from build123d import *

# Parameters (mm, degrees)
F1_DEPTH  = 38
F3_DEPTH  = 25
F4_DEPTH  = 38
F0_W      = 25
F0_H      = 10
F5_DEPTH  = 5
F6_DEPTH  = 10
F7_DEPTH  = 15
F0_W_2    = 5
F0_H_2    = 5
F8_DEPTH  = 38
F0_H_3    = 23
F9_DEPTH  = 32
F11_DEPTH = 15
F12_DEPTH = 20
F0_W_3    = 8.5
F13_DEPTH = 25
F14_DEPTH = 30
F15_DEPTH = 32


# Not quite as in the source:
# - the program builds the solid bodies; features that only make, move or delete a surface that nothing else refers to are left out


with BuildPart() as f1:
    # F0 (on Top) → F1 (new body)
    with BuildSketch(Plane.XY):
        Polygon((-33.5, 19), (-38.5, 19), (-38.5, -24), (-33.5, -24), (-33.5, -14), (-33.5, -4), align=None)
    extrude(amount=F1_DEPTH)

    # F2 (on face) → F3 (cut)
    with BuildSketch(Plane.YZ.offset(-33.5)):
        Polygon((-24, 38), (-24, 14), (19, 38), align=None)
    extrude(amount=-F3_DEPTH, mode=Mode.SUBTRACT)

    # F0 (on Top) → F4 (join)
    with BuildSketch(Plane.XY):
        Polygon((33.5, 19), (33.5, 24), (-38.5, 24), (-38.5, 19), (-33.5, 19), (-8.5, 19), (0, 19), (8.5, 19), align=None)
    extrude(amount=F4_DEPTH)

    # F0 (on Top) → F5 (join)
    with BuildSketch(Plane.XY):
        with Locations((-21, -19)):
            Rectangle(F0_W, F0_H)
    extrude(amount=F5_DEPTH)

    # F0 (on Top) → F6 (join)
    with BuildSketch(Plane.XY):
        Polygon((33.5, -14), (33.5, -4), (8.5, -4), (0, -4), (-8.5, -4), (-33.5, -4), (-33.5, -14), (-8.5, -14), align=None)
    extrude(amount=F6_DEPTH)

    # F0 (on Top) → F7 (join)
    with BuildSketch(Plane.XY):
        Polygon((38.5, -24), (38.5, -4), (33.5, -4), (33.5, -14), (33.5, -24), align=None)
    extrude(amount=F7_DEPTH)

    # F0 (on Top) → F8 (join)
    with BuildSketch(Plane.XY):
        with Locations((36, 21.5)):
            Rectangle(F0_W_2, F0_H_2)
    extrude(amount=F8_DEPTH)

    # F0 (on Top) → F9 (join)
    with BuildSketch(Plane.XY):
        with Locations((36, 7.5)):
            Rectangle(F0_W_2, F0_H_3)
    extrude(amount=F9_DEPTH)

    # F0 (on Top) → F11 (join)
    with BuildSketch(Plane.XY):
        Polygon((-8.5, -4), (-33.5, 19), (-33.5, -4), align=None)
    extrude(amount=F11_DEPTH)

    # F0 (on Top) → F12 (join)
    with BuildSketch(Plane.XY):
        Polygon((-8.5, 19), (-33.5, 19), (-8.5, -4), align=None)
    extrude(amount=F12_DEPTH)

    # F0 (on Top) → F13 (join)
    with BuildSketch(Plane.XY):
        with Locations((-4.25, 7.5)):
            Rectangle(F0_W_3, F0_H_3)
    extrude(amount=F13_DEPTH)

    # F0 (on Top) → F14 (join)
    with BuildSketch(Plane.XY):
        with Locations((4.25, 7.5)):
            Rectangle(F0_W_3, F0_H_3)
    extrude(amount=F14_DEPTH)

    # F0 (on Top) → F15 (join)
    with BuildSketch(Plane.XY):
        with Locations((21, 7.5)):
            Rectangle(F0_W, F0_H_3)
    extrude(amount=F15_DEPTH)


solid = f1.part
Can you work these out from the model? Positions are in its coordinate system, mm. A direction names the side the tool comes from. Round coordinates to 2 decimals unless told otherwise and drop trailing zeros. Loops run counter-clockwise (first coordinate to the right, second up) from the corner with the lowest first, then second, coordinate; pieces in that order, holes last. Notation, with made-up numbers: (1.5, 84.25) - (5.5, 84.25) arc R37 ccw to (5.5, 123.25) - close; hole circle Ø10 at (87.25, 0.25). An arc over 180 degrees is marked (long way). Write item = value, one per line. Start each with the question number.
(1) For P1, Ø11.5, axis at x = 18, y = 11, coming from the +Z side; P2, Ø4, axis at x = -21, y = 17.5, coming from the -Z side; P3, Ø5, axis at x = 30.5, z = 25, coming from the -Y side; P4, Ø8, axis at x = 6.5, z = 4, coming from the -Y side, each with a flat end and sliding along its axis, tell me the tip position at first contact or that it passes through.
(2) If we section it at D-D (y = -11.5): Please give me the cut outline in (x, z).
(3) If I drill on probe 1 along X at (y, z) = (14, 21.5); probe 2 along Y at (x, z) = (-26, 12.5); probe 3 along Z at (x, y) = (-7.5, -3), over which ranges is the centre line in solid material (lowest first)? Write a range as [from, to].
(4) If we section it at B-B (z = 12.5): Please give me the cut outline in (x, y), and give its area (3 significant figures).
(5) If we section it at C-C (x = -17.5): Please give me the cut outline in (y, z).
(6) If we mould it in two halves opening along X, with no side actions, what happens to faces 1 (the face through (-38.5, 6, 15)), 2 (the face through (10, -4, 21)), 3 (the face through (-21.175, 7.661, 17.465)), 4 (the face through (-1, 22, 38))? For each: released by +X, released by -X, zero draft, split by the parting line, or undercut.
(7) If we section it at A-A (y = -18.5): Please give me the cut outline in (x, z), and give its area (3 significant figures).
(8) For faces 5 (the face through (-8.5, -19, 2)), 6 (the face through (23, 8, 32)), 7 (the face through (-21, -19, 5)), which set-ups out of +Z, -Z, +X, -X, +Y, -Y let a thin tool reach every point of the face, with its end or its side?
Ans:
q1.P1 = 32
q1.P2 = 0
q1.P3 = -4
q1.P4 = -14
q2.outline = (-38.5, 0) - (38.5, 0) - (38.5, 15) - (33.5, 15) - (33.5, 10) - (-33.5, 10) - (-33.5, 20.98) - (-38.5, 20.98) - close
q3.probe_1 = [-38.5, -33.5], [-8.5, 38.5]
q3.probe_2 = [-4, 24]
q3.probe_3 = [0, 25]
q4.outline = (-38.5, -24) - (-33.5, -24) - (-33.5, -4) - (33.5, -4) - (33.5, -24) - (38.5, -24) - (38.5, 24) - (-38.5, 24) - close
q4.area = 2,360 mm²
q5.outline = (-24, 0) - (24, 0) - (24, 38) - (19, 38) - (19, 20) - (4.28, 20) - (4.28, 15) - (-4, 15) - (-4, 10) - (-14, 10) - (-14, 5) - (-24, 5) - close
q6.face_1 = released by -X
q6.face_2 = undercut
q6.face_3 = undercut
q6.face_4 = zero draft
q7.outline = (-38.5, 0) - (-8.5, 0) - (-8.5, 5) - (-33.5, 5) - (-33.5, 17.07) - (-38.5, 17.07) - close; (33.5, 0) - (38.5, 0) - (38.5, 15) - (33.5, 15) - close
q7.area = 285 mm²
q8.face_5 = +Z, -Z, -Y
q8.face_6 = +Z, +X, -Y
q8.face_7 = +Z, -Y
